from build123d import *

# Parameters (mm, degrees)
PAD_DEPTH   = 20
SKETCH002_W = 2
SKETCH002_H = 5.5
SKETCH004_W = 2
SKETCH004_H = 5.5
FILLET_R    = 1


with BuildPart() as part:
    # Sketch → Pad (new body)
    with BuildSketch(Plane.XY):
        with BuildLine():
            Line((0, 0), (5, 0))
            ThreePointArc((30.5, 0), (17.75, 12.75), (5, 0))
            Line((30.5, 0), (35.5, 0))
            Line((35.5, 0), (35.5, 80))
            Line((35.5, 80), (25.5, 80))
            ThreePointArc((10, 80), (17.75, 72.25), (25.5, 80))
            Line((10, 80), (0, 80))
            Line((0, 80), (0, 0))
        make_face()
    extrude(amount=PAD_DEPTH)

    # SubtractivePipe: sweep along a path in Sketch001
    with BuildLine(Plane.XY.offset(10)) as subtractivepipe_path:
        CenterArc((17.75, 0), 20, 0, 360)
    # Sketch002 → SubtractivePipe (sweep, cut)
    with BuildSketch(Plane.XZ):
        with Locations((37.5, 10)):
            Rectangle(SKETCH002_W, SKETCH002_H)
    sweep(path=subtractivepipe_path.line, mode=Mode.SUBTRACT)

    # SubtractivePipe001: sweep along a path in Sketch003
    with BuildLine(Plane.XY.offset(10)) as subtractivepipe001_path:
        CenterArc((17.75, 80), 20, 0, 360)
    # Sketch004 → SubtractivePipe001 (sweep, cut)
    with BuildSketch(Plane.XZ.offset(-80)):
        with Locations((37.5, 10)):
            Rectangle(SKETCH004_W, SKETCH004_H)
    sweep(path=subtractivepipe001_path.line, mode=Mode.SUBTRACT)

    # Fillet
    fillet_edges = [part.edges().sort_by_distance(p)[0] for p in [
        (35.5, 40, 20),
        (33, 0, 20),
        (17.75, 12.75, 20),
        (2.5, 0, 20),
        (0, 40, 20),
        (30.5, 80, 20),
        (17.75, 72.25, 20),
        (5, 80, 20),
        (0, 80, 10),
        (35.5, 80, 10),
        (35.5, 0, 10),
        (35.5, 40, 0),
        (5, 80, 0),
        (30.5, 80, 0),
        (17.75, 72.25, 0),
        (25.5, 80, 10),
        (10, 80, 10),
        (0, 40, 0),
        (0, 0, 10),
        (2.5, 0, 0),
        (17.75, 12.75, 0),
        (33, 0, 0),
        (30.5, 0, 10),
        (5, 0, 10),
    ]]
    fillet(fillet_edges, radius=FILLET_R)


solid = part.part
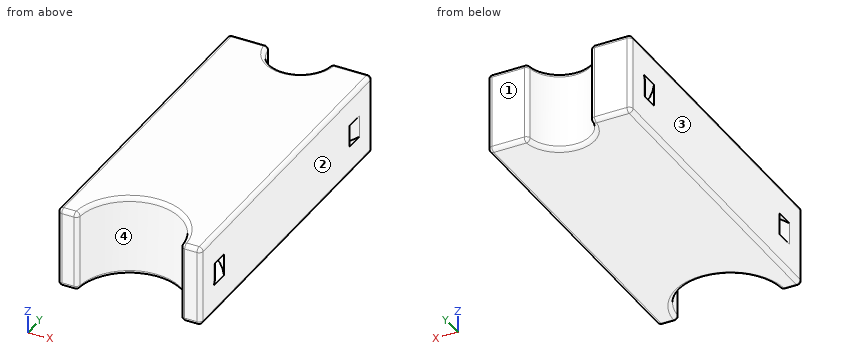
Input: part model. Units: mm. Frame: model coordinates. Face numbers are marked on the shaded views. Coordinates: 2 decimals unless noted, no trailing zeros. Order: outer loops, then holes, each group sorted by start corner. A loop starts at its lowest first (then second) coordinate and runs counter-clockwise, first axis right, second up. Notation, with made-up numbers: M 27,45 L 71,45 A30 ccw 71,83 Z; hole C -29,85 d6. An arc over 180 degrees is marked long. One line per question, with ' | ' between items.
Item 1: Ray query, line 1 along Y through (x, z) = (20.5, 11.25); line 2 along Y through (x, z) = (11, 9); line 3 along Z through (x, y) = (30, 15.5). Return the intervals inside material, ascending.
Geometry results:
line 1: y = 12.45 to 18.55, 20.57 to 59.43, 61.45 to 72.75 | line 2: y = 10.82 to 17.49, 19.62 to 60.38, 62.51 to 76.19 | line 3: z = 0 to 7.25, 12.75 to 20
Item 2: Section A-A (z = 2.5). Output: boundary loops of the cut face in (x, y).
Geometry results:
outline: M 0,1 A1 ccw 1,0 L 4.04,0 A1 ccw 5.03,0.93 A12.75 cw 30.47,0.93 A1 ccw 31.46,0 L 34.5,0 A1 ccw 35.5,1 L 35.5,79 A1 ccw 34.5,80 L 26.44,80 A1 ccw 25.45,79.11 A7.75 cw 10.05,79.11 A1 ccw 9.06,80 L 1,80 A1 ccw 0,79 Z
Item 3: Section B-B (x = 11.5). Give the number of separate pieces and of enclosed holes in the cut face, then the cut area to 3 significant figures.
Geometry results:
separate pieces: 1 | enclosed holes: 2 | area: 1,260 mm^2
Item 4: Draft query along X for the marked faces 1, 2, 3 and 4. Return one class per face: released by +X, released by -X, zero draft, split by the parting line, or undercut.
Geometry results:
face 1: zero draft | face 2: released by +X | face 3: released by -X | face 4: undercut
